Part model, mm, in its own coordinate system. A direction names the side the tool comes from. Coordinates: 2 decimals unless noted, no trailing zeros. Loops run counter-clockwise (first coordinate to the right, second up) from the corner with the lowest first, then second, coordinate; pieces in that order, holes last. Notation, with made-up numbers: (50.25, -29.75) -> (65.25, -29.75) arc R24 cw to (65.25, -14.75) -> close; hole circle Ø6 at (-19.75, -16). An arc over 180 degrees is marked (long way). Use one line per item in the form item = value. Start each with the question number.
(1) Drill centre lines: L1, parallel to Y at x = 0, z = 7; L2, parallel to X at y = 2.5, z = 15.25. Where is each one in solid material? Low to high. Write a range as [from, to].
(2) Band-saw the part on C-C on z = 7.25. Give the cut face in (x, y), then the cut area to 3 significant figures.
(3) Band-saw the part on B-B on x = 0. Give the cut face in (y, z).
(4) Pin check, flat tips, straight feed: P1, Ø2, axis at x = 2.5, y = 3.5, coming from the -Z side; P2, Ø1.5, axis at y = -0.5, z = 7, coming from the +X side; P3, Ø1, axis at y = -1.5, z = 3, coming from the +X side. Stop position of each tip, or through.
(5) Mould opens along X. For faces 3 (the flat face through (3, 0, 16)), 4 (the cylindrical face through (-3, 0, 7)), 5 (the flat face through (-0.8, 0, 15)), 6 (the flat face through (0.8, 0, 15)) say: +X half, -X half, draft (parallel to the pull), parting line (faces both ways), or undercut.
(6) Band-saw the part on A-A on y = 0. Give the cut face in (x, z).
(7) 3-axis set-ups, long thin cutter, end or side, ignore diameter. For faces 1 (the flat face through (0, 0, 0)), 2 (the flat face through (0, 0, 14.1)): which of +Z, -Z, +X, -X, +Y, -Y reach the whole face in a straight line?
(8) Band-saw the part on D-D on z = 14.5. Give the cut face in (x, y), then the cut area to 3 significant figures.
Solid Edge part; units mm, degrees
sketch "Sketch1" plane through (0, 0, 0) normal (0, -1, 0) x (1, 0, 0)
  line L0 (0, 0) -> (3, 0)
  line L1 (3, 0) -> (3, 13)
  line L2 (3, 13) -> (6, 16)
  line L3 (6, 16) -> (0, 16)
  line L4 (0, 16) -> (0, 0)
  dimension "D1" = 3
revolve "RevolvedProtrusion1" add sketch "Sketch1" angle 360 about axis through (0, 0, 54) along (0, 0, -1)
cosmetic_thread "Thread1"
sketch "Sketch2" plane through (0, 0, 0) normal (0, -1, 0) x (1, 0, 0)
  line L0 (-0.8, 16) -> (0.8, 16)
  line L1 (0.8, 16) -> (0.8, 14.1)
  line L2 (0.8, 14.1) -> (-0.8, 14.1)
  line L3 (-0.8, 14.1) -> (-0.8, 16)
  dimension "D1" = 0.8
  dimension "D2" = 0.8
extrude "Cutout1" cut sketch "Sketch2" along normal mid plane 73.4291
chamfer "Chamfer_1" distance 1 angle 45 1 edges at (-3, 0, 0)
properties part number "4" material "Fe 410 W"
A:
q1.L1 = [-3, 3]
q1.L2 = [-4.62, -0.8], [0.8, 4.62]
q2.outline = circle Ø6 at (0, 0)
q2.area = 28.3 mm²
q3.outline = (-4.1, 14.1) -> (-3, 13) -> (-3, 1) -> (-2, 0) -> (2, 0) -> (3, 1) -> (3, 13) -> (4.1, 14.1) -> close
q4.P1 = 13.3
q4.P2 = 3
q4.P3 = 2.83
q5.face_3 = draft
q5.face_4 = parting line
q5.face_5 = undercut
q5.face_6 = undercut
q6.outline = (-6, 16) -> (-3, 13) -> (-3, 1) -> (-2, 0) -> (2, 0) -> (3, 1) -> (3, 13) -> (6, 16) -> (0.8, 16) -> (0.8, 14.1) -> (-0.8, 14.1) -> (-0.8, 16) -> close
q7.face_1 = -Z, +X, -X, +Y, -Y
q7.face_2 = +Z, +Y, -Y
q8.outline = (-0.8, -4.43) -> (-0.8, 4.43) arc R4.5 ccw to start; (0.8, -4.43) arc R4.5 ccw to (0.8, 4.43) -> close
q8.area = 49.3 mm²
